The model under review builds one solid part; all positions refer to its coordinate system, in mm. A direction names the side the tool comes from. Coordinates: 2 decimals unless noted, no trailing zeros. Order: outer loops, then holes, each group sorted by start corner. A loop starts at its lowest first (then second) coordinate and runs counter-clockwise, first axis right, second up.
Autodesk Inventor part; units mm, degrees
ref_plane "YZ Plane" through (0, 0, 0) normal (1, 0, 0) x (0, 1, 0)
ref_plane "XZ Plane" through (0, 0, 0) normal (0, 1, 0) x (-1, 0, 0)
ref_plane "XY Plane" through (0, 0, 0) normal (0, 0, 1) x (1, 0, 0)
sketch "Sketch1" plane through (0, 0, 0) normal (1, 0, 0) x (0, 1, 0)
  line L0 (0, 0) -> (-20, 0)
  line L1 (-20, 0) -> (-20, -7)
  line L2 (-20, -7) -> (0, -7)
  line L3 (0, -7) -> (0, 0)
  line L4 (0, -7) -> (-7, -7)
  line L5 (-7, -7) -> (-7, -150)
  line L6 (-7, -150) -> (0, -150)
  line L7 (0, -150) -> (0, -7)
  dimension "d0" = 7
  dimension "d1" = 20
  dimension "d2" = 7
  dimension "d3" = 150
extrude "Extrusion1" add sketch "Sketch1" along normal blind 30
sketch "Sketch2" plane through (0, -7, -150) normal (0, -1, 0) x (1, 0, 0)
  line L0 (0, 0) -> (30, 0)
  circle A0 centre (15, 0) radius 15
  point P0 (0, 150)
extrude "Extrusion2" add sketch "Sketch2" along normal blind 80 and the other way blind 7
sketch "Sketch3" plane through (0, -20, -7) normal (0, 0, -1) x (-1, 0, 0)
  circle A0 centre (-7.5, 10) radius 2.25
  circle A1 centre (-22.5, 10) radius 2.25
  line L0 (0, 0) -> (-30, 0)
  line L1 (-30, 0) -> (-30, 13)
  point P0 (0, 20)
  dimension "d10" = 10
  dimension "d11" = 4.5
  dimension "d12" = 4.5
  dimension "d13" = 10
  dimension "d14" = 15
  dimension "d15" = 7.5
sketch "Sketch4" plane through (30, 0, 0) normal (1, 0, 0) x (0, 0, -1)
  line L0 (150, 0) -> (0, 0)
  line L1 (0, 0) -> (0, -20)
  line L2 (0, -20) -> (7, -20)
  line L3 (7, -20) -> (7, -7)
  line L4 (7, -7) -> (150, -7)
  line L5 (150, -7) -> (150, 0)
  line L6 (7, -20) -> (7, -7)
  line L7 (7, -20) -> (20, -7)
  line L8 (7, -7) -> (150, -7)
  line L9 (20, -7) -> (20, 0)
  dimension "d16" = 13
extrude "Extrusion3" add sketch "Sketch4" along normal blind 7 contours L9 L4 L3 L2 L1 L0 | L7 L3 L4
extrude "Extrusion4" cut sketch "Sketch3" against normal blind 7
sketch "Sketch5" plane through (0, 0, 0) normal (-1, 0, 0) x (0, 0, 1)
  line L0 (-150, 0) -> (0, 0)
  line L1 (-150, -7) -> (-150, 0)
  line L2 (-7, -7) -> (-150, -7)
  line L3 (-7, -20) -> (-7, -7)
  line L4 (0, -20) -> (-7, -20)
  line L5 (0, 0) -> (0, -20)
  line L6 (-7, -20) -> (-20, -7)
  line L7 (-7, -20) -> (-20, -7)
  line L8 (-20, 0) -> (-20, -7)
  line L9 (-20, -7) -> (-20, 0)
extrude "Extrusion5" add sketch "Sketch5" along normal blind 7 contours L0 L5 L4 L3 L2 L8 | L2 L3 L6
sketch "Sketch6" plane through (30, -20, -7) normal (0, 0, -1) x (-1, 0, 0)
  circle A0 centre (7.5, 10) radius 2.25
  circle A1 centre (22.5, 10) radius 2.25
  circle A2 centre (7.5, 10) radius 5.5
  circle A3 centre (22.5, 10) radius 5.5
  point P0 (30, 20)
  dimension "d23" = 11
  dimension "d24" = 11
extrude "Extrusion6" cut sketch "Sketch6" along normal blind 12
sketch "Sketch7" plane through (0, 0, 0) normal (-1, 0, 0) x (0, 0, 1)
  line L0 (-193.0937, 8.1233) -> (-158, 8.1233)
  line L1 (-158, 8.1233) -> (-158, -80)
  line L2 (-158, -80) -> (-193.0937, -80)
  line L3 (-193.0937, -80) -> (-193.0937, 8.1233)
  line L4 (-150, 0) -> (-165, 0)
  point P0 (0, 0)
  dimension "d27" = 80
  dimension "d28" = 7
extrude "Extrusion7" cut sketch "Sketch7" against normal blind 72
sketch "Sketch8" plane through (30, 0, -20) normal (0, 1, 0) x (1, 0, 0)
  line L0 (0, 145) -> (-118.3328, 145)
  line L1 (-118.3328, 145) -> (-118.3328, 116.9928)
  line L2 (-118.3328, 116.9928) -> (0, 116.9928)
  line L3 (0, 116.9928) -> (0, 145)
  line L4 (0, 130) -> (0, 0)
  arc A0 (-2.3114, 138) -> (-27.6886, 138) centre (-15, 130) ccw
  line L5 (-138.3328, 520) -> (-138.3328, -40)
  point P0 (-30, -20)
  dimension "d31" = 0
  dimension "d32" = 15
  dimension "d33" = 20
extrude "Extrusion8" add sketch "Sketch8" against normal blind 7
sketch "Sketch9" plane through (30, -7, -150) normal (0, -1, 0) x (1, 0, 0)
  line L0 (-118.3328, -22) -> (-111.3328, -22)
  line L1 (-111.3328, -22) -> (-111.3328, 20.0072)
  line L2 (-111.3328, 20.0072) -> (-118.3328, 20.0072)
  line L3 (-118.3328, 20.0072) -> (-118.3328, -22)
  line L4 (-118.3328, 13.0072) -> (-118.3328, -15)
  line L5 (-30, 13.0072) -> (-118.3328, 13.0072)
  line L6 (-118.3328, -15) -> (0, -15)
  point P0 (-30, 150)
  dimension "d36" = 7
  dimension "d37" = 0
  dimension "d38" = 7
  dimension "d39" = 7
extrude "Extrusion9" add sketch "Sketch9" along normal blind 13 and the other way blind 7
sketch "Sketch10" plane through (-81.3328, -20, -172) normal (0, 0, -1) x (-1, 0, 0)
  line L0 (7, 0) -> (0, 0)
  line L1 (0, 0) -> (-20, 20)
  line L2 (0, 20) -> (-81.3328, 20)
  line L3 (0, 20) -> (0, 0)
  line L4 (0, 13) -> (-111.3328, 13)
  line L5 (-13, 13) -> (-13, 20)
  dimension "d44" = 45
extrude "Extrusion10" add sketch "Sketch10" against normal blind 7 contours L1 L4 L3 | L5 L2 L3 L4
sketch "Sketch11" plane through (-88.3328, -20, -129.9928) normal (0, 0, 1) x (1, 0, 0)
  line L0 (7, 0) -> (7, 13)
  line L1 (20, 13) -> (27, 20)
  line L2 (7, 0) -> (20, 13)
  line L3 (20, 13) -> (20, 20)
  line L4 (0, 20) -> (20, 20)
  line L5 (7, 20) -> (7, 13)
  line L6 (7, 20) -> (7, 13)
  line L7 (7, 20) -> (20, 20)
  point P0 (88.3328, 20)
extrude "Extrusion11" add sketch "Sketch11" against normal blind 7
sketch "Sketch13" plane through (-81.3328, -20, -165) normal (1, 0, 0) x (0, 0, -1)
  circle A0 centre (-6.5, 10) radius 2.25
  circle A1 centre (-21.5, 10) radius 2.25
  line L0 (0, 0) -> (-28.0072, 0)
  line L1 (-158, 12.25) -> (-158, 7.75)
  line L2 (-158, 12.25) -> (-158, 7.75)
  line L3 (0, 0) -> (0, 13)
  line L4 (-28.0072, 13) -> (-28.0072, 0)
  point P0 (-165, 20)
  dimension "d49" = 10
  dimension "d50" = 10
  dimension "d51" = 15
  dimension "d52" = 6.5
  dimension "d53" = 6.5072
  dimension "d54" = 4.5
  dimension "d55" = 4.5
extrude "Extrusion12" cut sketch "Sketch13" against normal blind 7
sketch "Sketch15" plane through (-81.3328, -20, -165) normal (1, 0, 0) x (0, 0, -1)
  circle A0 centre (-6.5, 10) radius 2.25
  circle A1 centre (-6.5, 10) radius 5
  circle A2 centre (-21.5, 10) radius 2.25
  circle A3 centre (-21.5, 10) radius 5
  point P0 (-165, 20)
  dimension "d58" = 10
  dimension "d59" = 10
extrude "Extrusion13" cut sketch "Sketch15" along normal blind 20 contours A1 | A2 | A3
equation "\"d12\" = d11"
equation "\"d13\" = d10"
properties part number "SpoolHolder"
(1) Wall thickness on probe 1 along Y at (x, z) = (22.5, -3.5); probe 2 along X at (y, z) = (-6.5, -112); probe 3 along Z at (x, y) = (-7.5, -5): over which ranges is each line inside the solid? List them lowest first.
A:
probe 1: y = -20 to -12.25, -7.75 to 0
probe 2: x = 0 to 30
probe 3: z = -165 to -136.99
(2) Machinability: for faces 1 (the face through (7.6, -4.5, -12.9)), 2 (the face through (-68.333, -4, -133)), 3 (the face through (-7, -8, -8)), 4 (the face through (-84.784, -9.324, -145.646)), 5 (the face through (7.79, -7.77, -3.55)), which of the approach directions +Z, -Z, +X, -X, +Y, -Y give a long, thin tool a straight path to every point of the face, cutting with its end or side? Answer none if there is none.
A:
face 1: -Y
face 2: +Z, +Y, -Y
face 3: +Z, -X, +Y, -Y
face 4: -X
face 5: +Z
(3) We need section D-D, the plane y = -29. Write out the cut boundary in (x, z), and give its area (3 significant figures).
A:
outline: (2.31, -158) - (27.69, -158) arc R15 ccw (long way) to start
area: 582 mm2
(4) For pin 1 Ø10.5 at (x, y) = (-77.5, -12.5) entering from +Z; pin 2 Ø12 at (x, z) = (-60, -150.5) entering from -Y; pin 3 Ø3.5 at (x, y) = (7.5, -10) entering from +Z; pin 4 Ø1.5 at (y, z) = (-22, -130.5) entering from -X, all flat-tipped, find the tip position at first contact; note any pin that passes through.
A:
pin 1: stops at z = -129.99
pin 2: stops at y = -7
pin 3: stops at z = -136.15
pin 4: passes through
(5) We need section A-A, the plane y = -10. Count the separate pieces of the cut face and the enclosed holes in it, and give its area (3 significant figures).
A:
separate pieces: 7
enclosed holes: 0
area: 1,340 mm2
(6) We need section B-B, the plane x = 22.5. Write out the cut boundary in (y, z).
A:
outline: (-87, -162.99) - (-80, -162.99) - (-80, -158) - (-7, -158) - (-7, -165) - (0, -165) - (0, 0) - (-7.75, 0) - (-7.75, -7) - (-4.5, -7) - (-4.5, -19) - (-7, -19) - (-7, -137.01) - (-87, -137.01) - close; (-20, -7) - (-12.25, -7) - (-12.25, 0) - (-20, 0) - close
(7) We need section C-C, the plane z = -143.5. Write out the cut boundary in (x, y), and give its area (3 significant figures).
A:
outline: (-88.33, -20) - (-81.33, -20) - (-81.33, -12.25) - (-88.33, -12.25) - close; (-88.33, -7.75) - (-81.33, -7.75) - (-81.33, -5) - (-61.33, -5) - (-61.33, -7) - (1.48, -7) - (1.48, -87) - (28.52, -87) - (28.52, -7) - (30, -7) - (30, 0) - (-88.33, 0) - close
area: 3,010 mm2
(8) Draft analysis for pull direction Y (two halves, no side actions). For faces 6 (the face through (30, -3, -91)), 7 (the face through (-84.784, -9.324, -160.646)), 8 (the face through (22.6, -4.5, -12.9)), state which applies: released by +Y, released by -Y, zero draft, split by the parting line, or undercut.
A:
face 6: zero draft
face 7: undercut
face 8: released by -Y
